CAD build for the part. Positions are in the model's coordinates, mm. A direction names the side the tool comes from. Give positions to 0.01 mm unless a question says otherwise; leave off trailing zeros. Loops run counter-clockwise (first coordinate to the right, second up) from the corner with the lowest first, then second, coordinate; pieces in that order, holes last. Notation, with made-up numbers: M 61,33 L 90,33 A8 ccw 90,40 Z; hole C -29,-33 d2. An arc over 180 degrees is marked long. One line per question, with ' | ' between items.
```python
from build123d import *

# Parameters (mm, degrees)
PAD002_DEPTH = 16
POCKET_DEPTH = 2.5
FILLET001_R  = 1


with BuildPart() as part:
    # Sketch003 → Pad002 (new body)
    with BuildSketch(Plane.XY):
        with BuildLine():
            Line((7.15, -7.803847), (-7.15, -7.803847))
            Line((-7.15, -7.803847), (-7.15, 3))
            ThreePointArc((-2.95, 7.2), (-5.919848, 5.969848), (-7.15, 3))
            Line((-2.95, 7.2), (2.95, 7.2))
            ThreePointArc((7.15, 3), (5.919848, 5.969848), (2.95, 7.2))
            Line((7.15, 3), (7.15, -7.803847))
        make_face()
    extrude(amount=PAD002_DEPTH)

    # Sketch004 → Pocket (cut)
    with BuildSketch(Plane.XY.offset(2.5)):
        with BuildLine():
            ThreePointArc((-2.95, 5.2), (-4.505635, 4.555635), (-5.15, 3))
            Line((-5.15, 1), (-5.15, 3))
            ThreePointArc((-5.15, -0.6), (-4.75, 0.2), (-5.15, 1))
            Line((-5.15, -7.803847), (-5.15, -0.6))
            Line((5.15, -7.803847), (-5.15, -7.803847))
            Line((5.15, -0.6), (5.15, -7.803847))
            ThreePointArc((5.15, 1), (4.75, 0.2), (5.15, -0.6))
            Line((5.15, 3), (5.15, 1))
            ThreePointArc((5.15, 3), (4.505635, 4.555635), (2.95, 5.2))
            Line((-2.95, 5.2), (2.95, 5.2))
        make_face()
    extrude(amount=POCKET_DEPTH, mode=Mode.SUBTRACT)

    # Fillet001
    fillet001_edges = [part.edges().sort_by_distance(p)[0] for p in [
        (-5.919848, 5.969848, 0),
        (-5.919848, 5.969848, 16),
        (-7.15, -7.803847, 8),
        (7.15, -7.803847, 8),
        (0, -7.803847, 16),
        (0, -7.803847, 0),
    ]]
    fillet(fillet001_edges, radius=FILLET001_R)


solid = part.part
```
Item 1: 3-axis set-ups, long thin cutter, end or side, ignore diameter. For faces 5 (the flat face through (0, 0, 16)), 6 (the flat face through (0, 5.2, 4)), 7 (the flat face through (5.15, 2, 4)): which of +Z, -Z, +X, -X, +Y, -Y reach the whole face in a straight line?
Conclusion:
face 5: +Z, +X, -X, +Y, -Y | face 6: -Y | face 7: none
Item 2: Drill centre lines: line 1 along Z through (x, y) = (0.75, -2); line 2 along X through (y, z) = (-1.25, 3.5); line 3 along X through (y, z) = (3.75, 4). Where is each one in solid material? Low to high. Write a range as [from, to].
Conclusion:
line 1: [0, 2.5], [5, 16] | line 2: [-7.15, -5.15], [5.15, 7.15] | line 3: [-7.08, -5.02], [5.02, 7.08]
Item 3: Saw through at C-C on z = 2.25. Give the cut face in (x, y).
Conclusion:
outline: M -7.15,-6.8 A1 ccw -6.15,-7.8 L 6.15,-7.8 A1 ccw 7.15,-6.8 L 7.15,3 A4.2 ccw 2.95,7.2 L -2.95,7.2 A4.2 ccw -7.15,3 Z
Item 4: Mould opens along Y. For faces 1 (the cylindrical face through (-0.041, 6.899, 0.285)), 2 (the cylindrical face through (4.52, 4.54, 3.73)), 3 (the flat face through (0, -7.804, 9)), 4 (the flat face through (7.15, -2, 8)) say: pulls with the +Y half, pulls with the -Y half, needs draft (parallel to the pull), parting line crosses it, or undercut.
Conclusion:
face 1: pulls with the +Y half | face 2: undercut | face 3: pulls with the -Y half | face 4: needs draft
Item 5: Saw through at A-A on y = -5. Give the cut face in (x, z), and give its area (3 significant figures).
Conclusion:
outline: M -7.15,1 A1 ccw -6.15,0 L 6.15,0 A1 ccw 7.15,1 L 7.15,15 A1 ccw 6.15,16 L -6.15,16 A1 ccw -7.15,15 Z; hole M -5.15,2.5 L 5.15,2.5 L 5.15,5 L -5.15,5 Z | area: 202 mm²
Item 6: Drop a flat-ended pin along its axis: P1, Ø6, axis at x = -4, z = 14, coming from the +Y side. Give the stop position or say it passes through.
Conclusion:
P1: y = 7.2
Item 7: Saw through at B-B on x = 1.25. Give the cut face in (y, z), and give its area (3 significant figures).
Conclusion:
outline: M -7.8,1 A1 ccw -6.8,0 L 6.2,0 A1 ccw 7.2,1 L 7.2,15 A1 ccw 6.2,16 L -6.8,16 A1 ccw -7.8,15 L -7.8,5 L 5.2,5 L 5.2,2.5 L -7.8,2.5 Z | area: 207 mm²
